Geometry: see drawing. Coordinates: mm, zero at the bounding-box minimum. A direction names the side the tool comes from. Coordinates: 2 decimals unless noted, no trailing zeros. Loops run counter-clockwise (first coordinate to the right, second up) from the corner with the lowest first, then second, coordinate; pieces in that order, holes last. Notation, with made-up numbers: (58, 11.5) -> (69, 11.5) arc R33 ccw to (69, 49.5) -> close; hole circle Ø2 at (40, 20). An arc over 180 degrees is marked (long way). One line per item, written item: value. Start each with the question number.
Item 1: Section query A-A on x = 13.75. Return loops of the section in (y, z).
Item 2: Section query D-D on x = 20.75. Return loops of the section in (y, z), then the cut area to 3 significant figures.
Item 3: Contact query for flat-ended pins moving along their axis: pin 1 Ø1.5 at (y, z) = (13.5, 5.5) entering from -X (1 decimal); pin 2 Ø1.5 at (y, z) = (47.5, 11.5) entering from -X (1 decimal); pin 3 Ø6 at (y, z) = (32, 4.5) entering from -X. Output: stop coordinate, or through.
Item 4: Section query B-B on y = 53.5. Return loops of the section in (x, z), then the cut area to 3 significant figures.
Item 5: Ray query, probe 1 along Y at (x, z) = (22, 7); probe 2 along Z at (x, y) = (2.25, 42.5) (1 decimal); probe 3 along Z at (x, y) = (1.75, 29.5) (1 decimal). Return the intervals inside material, ascending. Write a range as from..to.
Item 6: Set-up query: the marked faces 1 and 2. Return all of +Z, -Z, +X, -X, +Y, -Y with unobstructed straight access to the full face (end or side cutting, diameter ignored); none if empty.
Item 7: Section query C-C on z = 5. Return loops of the section in (x, y) (1 decimal).
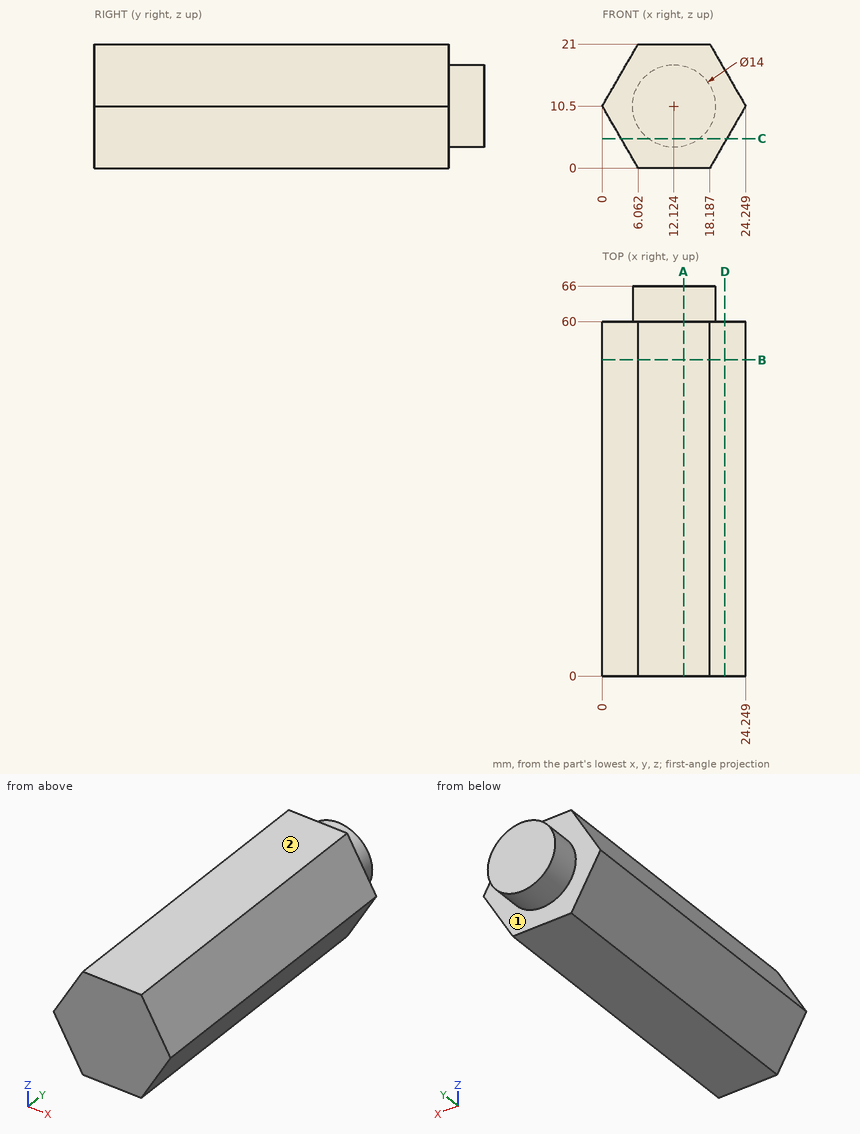
Reply:
1. outline: (0, 0) -> (60, 0) -> (60, 3.69) -> (66, 3.69) -> (66, 17.31) -> (60, 17.31) -> (60, 21) -> (0, 21) -> close
2. outline: (0, 4.44) -> (60, 4.44) -> (60, 16.56) -> (0, 16.56) -> close
2. area: 727 mm²
3. pin 1: stops at x = 2.5
3. pin 2: stops at x = 0.1
3. pin 3: stops at x = 1.73
4. outline: (0, 10.5) -> (6.06, 0) -> (18.19, 0) -> (24.25, 10.5) -> (18.19, 21) -> (6.06, 21) -> close
4. area: 382 mm²
5. probe 1: y = 0..60
5. probe 2: z = 6.6..14.4
5. probe 3: z = 7.5..13.5
6. face 1: +Y
6. face 2: +Z, +X, -X, +Y, -Y
7. outline: (3.2, 0) -> (21.1, 0) -> (21.1, 60) -> (16.5, 60) -> (16.5, 66) -> (7.8, 66) -> (7.8, 60) -> (3.2, 60) -> close
